Geometry: final body of the model. Coordinates: model frame, mm. A direction names the side the tool comes from. Round coordinates to 2 decimals unless told otherwise and drop trailing zeros. Loops run counter-clockwise (first coordinate to the right, second up) from the corner with the lowest first, then second, coordinate; pieces in that order, holes last. Notation, with made-up numbers: (35, -40) - (83, -40) arc R24 cw to (83, -1) - close; hole circle Ø9 at (44.5, 89). An arc over 180 degrees is marked (long way). Write item = value, one per line. Start each with the question number.
Item 1: Draft query along X for faces 1 (the flat face through (-11, 19.9, 16.9)), 2 (the conical face through (7.9, 20.5, 11)), 3 (the cylindrical face through (-0.15, 21.55, 18.96)). Return one class per face: pulls with the +X half, pulls with the -X half, needs draft (parallel to the pull), parting line crosses it, or undercut.
Item 2: Section A-A (y = 0). Return loops of the section in (x, z), plus the area to 3 significant figures.
Item 3: Line query: line 1 (Y direction, x = 0, z = 1.2); line 2 (X direction, y = 7, z = 3); line 3 (Z direction, x = 9.5, y = -7). Output: solid intervals per line, ascending. Write a range as from..to.
Item 4: Section C-C (y = -17). Return loops of the section in (x, z) (3 decimals), plus the area to 3 significant figures.
Item 5: Section B-B (x = 4). Count the separate pieces of the cut face and the enclosed holes in it, plus the area to 3 significant figures.
Item 6: Access query for faces 4 (the flat face through (20, 0, 6)), 5 (the conical face through (-7.9, 20.5, 11.2)), 6 (the cylindrical face through (-20.5, -15.45, 2.49)), 7 (the flat face through (-20, 14, 16)), 8 (the flat face through (19.726, -17, 2)). Directions: +Z, -Z, +X, -X, +Y, -Y. A direction counts if a zero-diameter tool reaches every point of the face in a straight line with its end or side. Return the directions, or none.
Item 7: First-contact query: pin 1 (8 mm diameter, centred on x = -7.5, y = 15.5, fed in from +Z); pin 2 (23 mm diameter, centred on x = 0, y = 0, fed in from +Z); pin 3 (3.5 mm diameter, centred on y = 21.5, z = 18, fed in from +X); pin 4 (1 mm diameter, centred on x = 5, z = 9, fed in from +Y). Flat tips, straight axial feed; report the tip coordinate or a pass-through.
from build123d import *

# Parameters (mm, degrees)
SKETCH1_W                = 38.5
SKETCH1_H                = 38
SKETCH1_R                = 10
BOSS_EXTRUDE1_DEPTH      = 2
BOSS_EXTRUDE2_DEPTH      = 14
BOSS_EXTRUDE2_DEPTH_BACK = 2
CUT_EXTRUDE1_REACH       = 50.345
SKETCH3_W                = 10
SKETCH3_H                = 2.5
CUT_EXTRUDE2_DEPTH       = 47.384938288
CUT_EXTRUDE2_DRAFT       = 15
FILLET1_R                = 1
BOSS_EXTRUDE3_DEPTH      = 11
BOSS_EXTRUDE3_DEPTH_BACK = 11
SKETCH7_R                = 0.825
SKETCH8_R                = 1.625
CUT_EXTRUDE3_DEPTH       = 1.524


with BuildPart() as part:
    # Sketch1 → Boss-Extrude1 (new body)
    with BuildSketch(Plane.XY):
        Rectangle(SKETCH1_W, SKETCH1_H)
        Circle(SKETCH1_R, mode=Mode.SUBTRACT)
    extrude(amount=BOSS_EXTRUDE1_DEPTH)

    # Sketch2 → Boss-Extrude2 (add, two sides: drawn at the far end of the back side and taken through both)
    with BuildSketch(Plane.XY.offset(2).offset(-BOSS_EXTRUDE2_DEPTH_BACK)):
        Polygon((-21.25, -19), (-19.25, -19), (-19.25, 19), (19.25, 19), (19.25, -19), (21.25, -19), (21.25, 21), (-21.25, 21), align=None)
    extrude(amount=BOSS_EXTRUDE2_DEPTH + BOSS_EXTRUDE2_DEPTH_BACK)

    # Sketch3 → Cut-Extrude1 (cut, up to next)
    with BuildSketch(Plane(origin=(-19.25, 0, 0), x_dir=(0, 0, -1), z_dir=(1, 0, 0)), mode=Mode.PRIVATE) as cut_extrude1_sk1:
        with Locations((-11, 0)):
            Rectangle(SKETCH3_W, SKETCH3_H)
    cut_extrude1_tool1 = extrude(cut_extrude1_sk1.sketch, amount=-CUT_EXTRUDE1_REACH, mode=Mode.PRIVATE) & part.part
    cut_extrude1 = cut_extrude1_tool1.solids().sort_by_distance((-19.25, 0, 11))[0]
    add(cut_extrude1, mode=Mode.SUBTRACT)

    # Mirror1: Cut-Extrude1 across plane
    add(cut_extrude1.mirror(Plane(origin=(0, 0, 0), x_dir=(0, 0, 1), z_dir=(1, 0, 0))), mode=Mode.SUBTRACT)


with BuildPart() as cut_extrude2_tool:
    # Sketch5 → Cut-Extrude2 (with draft: the straight prism first)
    with BuildSketch(Plane.XZ.offset(-19)):
        with BuildLine():
            ThreePointArc((-5, 13.591034656), (-7.5, 11.091034656), (-5, 8.591034656))
            Line((-5, 8.591034656), (5, 8.591034656))
            ThreePointArc((5, 8.591034656), (7.5, 11.091034656), (5, 13.591034656))
            Line((5, 13.591034656), (-5, 13.591034656))
        make_face()
    extrude(amount=-CUT_EXTRUDE2_DEPTH)
    # Cut-Extrude2: the draft: its side faces are tilted about the plane it starts from
    cut_extrude2_sides = [cut_extrude2_tool.faces().sort_by_distance(p)[0] for p in [
        (0, 42.692469144, 13.591034656),
        (-7.5, 42.692469144, 11.091034656),
        (0, 42.692469144, 8.591034656),
        (7.5, 42.692469144, 11.091034656),
    ]]
    draft(cut_extrude2_sides, Plane.XZ.offset(-19), CUT_EXTRUDE2_DRAFT)


with BuildPart() as part_1:
    add(part.part)

    # Cut-Extrude2: cut by cut_extrude2_tool
    add(cut_extrude2_tool.part, mode=Mode.SUBTRACT)

    # Fillet1
    fillet1_edges = [part_1.edges().sort_by_distance(p)[0] for p in [
        (-7.5, 19, 11.091034656),
        (0, 19, 8.591034656),
        (7.5, 19, 11.091034656),
        (0, 19, 13.591034656),
    ]]
    fillet(fillet1_edges, radius=FILLET1_R)

    # Sketch7 → Boss-Extrude3 (add, two sides: drawn at the far end of the back side and taken through both)
    with BuildSketch(Plane(origin=(0, 0, 0), x_dir=(0, 0, -1), z_dir=(1, 0, 0)).offset(-BOSS_EXTRUDE3_DEPTH_BACK)):
        with BuildLine():
            Line((-17.625, 19), (-16, 19))
            Line((-16, 19), (-16, 21))
            ThreePointArc((-16, 21), (-16.073732036, 21.14399831), (-16.142494793, 21.290434678))
            ThreePointArc((-16.142494793, 21.290434678), (-18.989176739, 21.507976118), (-17.625, 19))
        make_face()
        with Locations((-17.625, 20.625)):
            Circle(SKETCH7_R, mode=Mode.SUBTRACT)
    extrude(amount=BOSS_EXTRUDE3_DEPTH + BOSS_EXTRUDE3_DEPTH_BACK)

    # Sketch8 → Cut-Extrude3 (cut)
    with BuildSketch(Plane(origin=(21.25, 0, 0), x_dir=(0, 0, -1), z_dir=(1, 0, 0))):
        with Locations(Location((-2, -17, 0), (0, 0, 90))):
            Circle(SKETCH8_R)
    cut_extrude3 = extrude(amount=-CUT_EXTRUDE3_DEPTH, mode=Mode.SUBTRACT)

    # Mirror2: Cut-Extrude3 across plane
    add(cut_extrude3.mirror(Plane(origin=(0, 0, 0), x_dir=(0, 0, 1), z_dir=(1, 0, 0))), mode=Mode.SUBTRACT)


solid = part_1.part
Taken from the geometry:
q1.face_1 = pulls with the -X half
q1.face_2 = undercut
q1.face_3 = needs draft
q2.outline = (-21.25, 0) - (-10, 0) - (-10, 2) - (-19.25, 2) - (-19.25, 6) - (-21.25, 6) - close; (10, 0) - (21.25, 0) - (21.25, 6) - (19.25, 6) - (19.25, 2) - (10, 2) - close
q2.area = 61.0 mm^2
q3.line_1 = -19..-10, 10..21
q3.line_2 = -21.25..-19.25, 19.25..21.25
q3.line_3 = 0..2
q4.outline = (-21.25, 0) - (21.25, 0) - (21.25, 0.375) - (19.726, 0.375) - (19.726, 3.625) - (21.25, 3.625) - (21.25, 16) - (19.25, 16) - (19.25, 2) - (-19.25, 2) - (-19.25, 16) - (-21.25, 16) - (-21.25, 3.625) - (-19.726, 3.625) - (-19.726, 0.375) - (-21.25, 0.375) - close
q4.area = 131 mm^2
q5.separate_pieces = 3
q5.enclosed_holes = 1
q5.area = 66.2 mm^2
q6.face_4 = +Z, +X, -X
q6.face_5 = +Y
q6.face_6 = -X
q6.face_7 = +Z, -X, +Y, -Y
q6.face_8 = +X
q7.pin_1 = 18.8
q7.pin_2 = 2
q7.pin_3 = 11
q7.pin_4 = through
